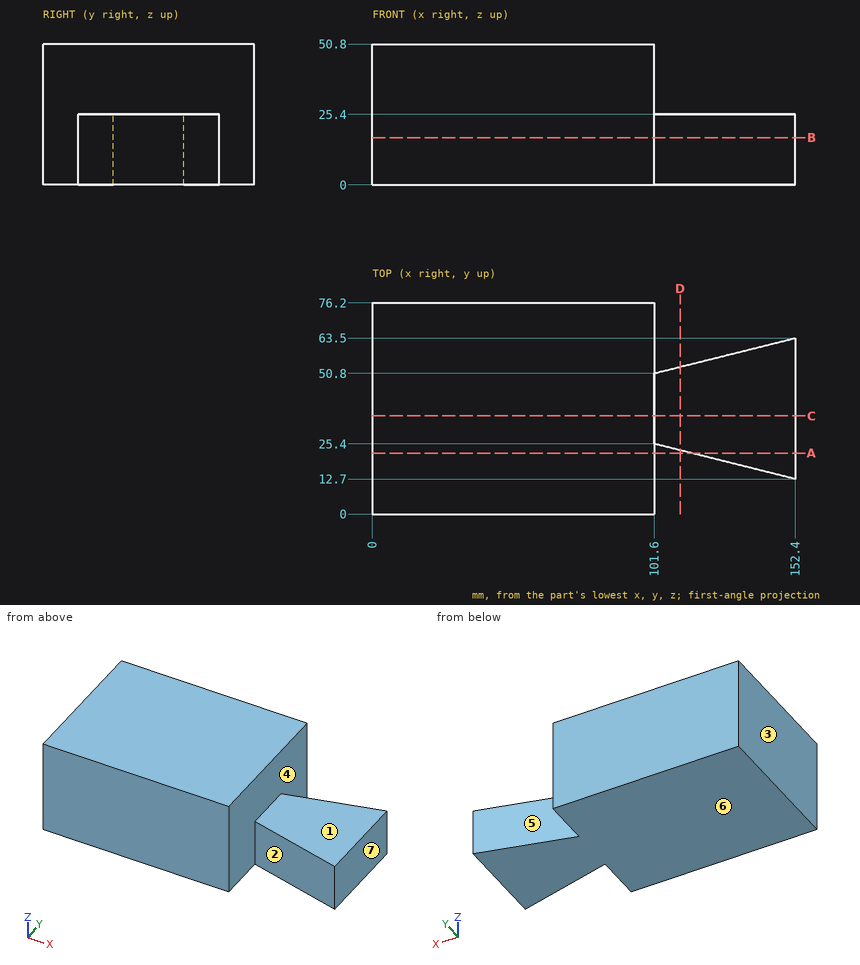
Geometry: see drawing. Coordinates: mm, zero at the bounding-box minimum. A direction names the side the tool comes from. Coordinates: 2 decimals unless noted, no trailing zeros. Order: outer loops, then holes, each group sorted by start corner. A loop starts at its lowest first (then second) coordinate and runs counter-clockwise, first axis right, second up. Notation, with made-up numbers: M 64.25,9 L 69.25,9 A29 ccw 69.25,44 Z; hole C 40.25,5.25 d2. An arc over 180 degrees is marked long. Answer in a Markdown table with one row per item. Add a question column.
Q1. Section query B-B on z = 17. Return the cut outline in (x, y), and give its area (3 significant figures).
Q2. Mould query, pull axis X, two halves, no side actions, for the marked faces 5, 6 and 7. Classes: released by +X, released by -X, zero draft, split by the parting line, or undercut.
Q3. Line query: L1, parallel to Z at x = 108.5, y = 40.5; L2, parallel to X at y = 11.5, z = 21.5; L3, parallel to Y at x = 144.5, z = 11.5 (3 decimals). Output: solid intervals per line, ascending.
Q4. Section query C-C on y = 35.5. Return the cut outline in (x, z).
Q5. Section query D-D on x = 111. Return the cut outline in (y, z), and give its area (3 significant figures).
Q6. Contact query for a flat-ended pin moving along its axis: P1, Ø12, axis at x = 116.5, z = 22, coming from the +Y side (3 decimals). Output: stop coordinate, or through.
Q7. Section query A-A on y = 22. Return the cut outline in (x, z).
Q8. Reachability of the marked faces 1, 2, 3 and 4 from +Z, -Z, +X, -X, +Y, -Y: full face, straight path, thin tool, end or side. Return the list, or none.
Completed:
| question | item | result |
|---|---|---|
| 1 | outline | M 0,0 L 101.6,0 L 101.6,25.4 L 152.4,12.7 L 152.4,63.5 L 101.6,50.8 L 101.6,76.2 L 0,76.2 Z |
| 1 | area | 9,680 mm2 |
| 2 | face 5 | undercut |
| 2 | face 6 | zero draft |
| 2 | face 7 | released by +X |
| 3 | L1 | z = 0 to 25.4 |
| 3 | L2 | x = 0 to 101.6 |
| 3 | L3 | y = 14.675 to 61.525 |
| 4 | outline | M 0,0 L 152.4,0 L 152.4,25.4 L 101.6,25.4 L 101.6,50.8 L 0,50.8 Z |
| 5 | outline | M 23.05,0 L 53.15,0 L 53.15,25.4 L 23.05,25.4 Z |
| 5 | area | 765 mm2 |
| 6 | P1 | stops at y = 56.025 |
| 7 | outline | M 0,0 L 101.6,0 L 101.6,50.8 L 0,50.8 Z; M 115.2,0 L 152.4,0 L 152.4,25.4 L 115.2,25.4 Z |
| 8 | face 1 | +Z, +X, +Y, -Y |
| 8 | face 2 | +Z, -Z, -Y |
| 8 | face 3 | +Z, -Z, -X, +Y, -Y |
| 8 | face 4 | +Z |
